```python
from build123d import *

# Parameters (mm, degrees)
F1_DEPTH = 152.4
F2_R     = 8.73125
F3_DEPTH = 76.201
F4_R     = 6.35
F5_DEPTH = 101.601


with BuildPart() as f1:
    # F0 (on Front) → F1 (new body, symmetric)
    with BuildSketch(Plane.XZ):
        with BuildLine():
            Line((3.175, 76.2), (0, 76.2))
            Line((0, 76.2), (0, 0))
            Line((0, 0), (101.6, 0))
            Line((101.6, 0), (101.6, 3.175))
            ThreePointArc((101.6, 3.175), (100.6700640303, 5.4200640303), (98.425, 6.35))
            Line((98.425, 6.35), (9.525, 6.35))
            ThreePointArc((9.525, 6.35), (7.2799359697, 7.2799359697), (6.35, 9.525))
            Line((6.35, 9.525), (6.35, 73.025))
            ThreePointArc((6.35, 73.025), (5.4200640303, 75.2700640303), (3.175, 76.2))
        make_face()
    extrude(amount=F1_DEPTH, both=True)

    # F2 (on face) → F3 (cut, through all)
    with BuildSketch(Plane(origin=(0, 0, 0), x_dir=(1, 0, 0), z_dir=(0, 0, -1))):
        with Locations((50.8, 50.8)):
            Circle(F2_R)
        with Locations((50.8, -50.8)):
            Circle(F2_R)
    extrude(amount=-F3_DEPTH, mode=Mode.SUBTRACT)

    # F4 (on face) → F5 (cut, through all)
    with BuildSketch(Plane(origin=(0, 0, 0), x_dir=(0, -1, 0), z_dir=(-1, 0, 0))):
        with Locations((-114.3, 38.1)):
            Circle(F4_R)
        with Locations((114.3, 38.1)):
            Circle(F4_R)
    extrude(amount=-F5_DEPTH, mode=Mode.SUBTRACT)


solid = f1.part
```
Source: CAD feature listing. Evaluate the final solid. Frame: model axes, mm. A direction names the side the tool comes from. Round coordinates to 2 decimals unless told otherwise and drop trailing zeros. Loops run counter-clockwise (first coordinate to the right, second up) from the corner with the lowest first, then second, coordinate; pieces in that order, holes last. Notation, with made-up numbers: M -14.5,-33.5 L 11.5,-33.5 A23 ccw 11.5,-11.5 Z; hole C -17,48 d4. An arc over 180 degrees is marked long. Use a Markdown table: item, result. Add a question column.
1. Cut plane B-B, the plane y = -114.3. Output: boundary loops of the cut face in (x, z) (3 decimals).
2. Cut plane C-C, the plane y = -50.8. Output: boundary loops of the cut face in (x, z) (3 decimals), and give its area (3 significant figures).
3. Cut plane A-A, the plane x = 50.8. Output: boundary loops of the cut face in (y, z), and give its area (3 significant figures).
4. Ray query, line 1 along Y through (x, z) = (50.8, 3.5); line 2 along Y through (x, z) = (1, 38); line 3 along Z through (x, y) = (3, -114). Return the intervals inside material, ascending. Write a range as [from, to].
5. Cut plane D-D, the plane x = 68.5. Output: boundary loops of the cut face in (y, z), and give its area (3 significant figures).
6. Contact query for flat-ended pins moving along their axis: pin 1 (2 mm diameter, centred on x = 55, y = -32.5, fed in from +Z); pin 2 (3 mm diameter, centred on y = -69, z = 43.5, fed in from +X). Output: stop coordinate, or through.
7. Pull-direction query (Z, two-part tool) for faces 3 (the cylindrical face through (3.131, 111.37, 32.466)), 4 (the flat face through (50, -2, 0)), 5 (the cylindrical face through (3.13, -109.26, 34.24)), 6 (the flat face through (28, -152.4, 4)); classes: +Z half, -Z half, draft (parallel to the pull), parting line (faces both ways), or undercut.
8. Set-up query: faces 1 (the flat face through (6.35, -2, 41)), 2 (the cylindrical face through (42.077, -51.184, 3.131)). Return all of +Z, -Z, +X, -X, +Y, -Y with unobstructed straight access to the full face (end or side cutting, diameter ignored); none if empty.
Solution:
| question | item | result |
|---|---|---|
| 1 | outline | M 0,0 L 101.6,0 L 101.6,3.175 A3.175 ccw 98.425,6.35 L 9.525,6.35 A3.175 cw 6.35,9.525 L 6.35,31.75 L 0,31.75 Z; M 0,44.45 L 6.35,44.45 L 6.35,73.025 A3.175 ccw 3.175,76.2 L 0,76.2 Z |
| 2 | outline | M 0,0 L 42.069,0 L 42.069,6.35 L 9.525,6.35 A3.175 cw 6.35,9.525 L 6.35,73.025 A3.175 ccw 3.175,76.2 L 0,76.2 Z; M 59.531,0 L 101.6,0 L 101.6,3.175 A3.175 ccw 98.425,6.35 L 59.531,6.35 Z |
| 2 | area | 976 mm2 |
| 3 | outline | M -152.4,0 L -59.53,0 L -59.53,6.35 L -152.4,6.35 Z; M -42.07,0 L 42.07,0 L 42.07,6.35 L -42.07,6.35 Z; M 59.53,0 L 152.4,0 L 152.4,6.35 L 59.53,6.35 Z |
| 3 | area | 1,710 mm2 |
| 4 | line 1 | y = [-152.4, -59.53], [-42.07, 42.07], [59.53, 152.4] |
| 4 | line 2 | y = [-152.4, -120.65], [-107.95, 107.95], [120.65, 152.4] |
| 4 | line 3 | z = [0, 31.76], [44.44, 76.2] |
| 5 | outline | M -152.4,0 L 152.4,0 L 152.4,6.35 L -152.4,6.35 Z |
| 5 | area | 1,940 mm2 |
| 6 | pin 1 | stops at z = 6.35 |
| 6 | pin 2 | stops at x = 6.35 |
| 7 | face 3 | undercut |
| 7 | face 4 | -Z half |
| 7 | face 5 | undercut |
| 7 | face 6 | draft |
| 8 | face 1 | +Z, +X, +Y, -Y |
| 8 | face 2 | +Z, -Z |
